```python
from build123d import *

# Parameters (mm, degrees)
IZIM1_R                     = 2
Y_KSEKLIK_EKSTR_ZYON1_DEPTH = 2.5
KES_EKSTR_ZYON1_START       = -2.5
IZIM2_R                     = 2
KES_EKSTR_ZYON1_DEPTH       = 2.5


with BuildPart() as part:
    # Çizim1 → Yükseklik-Ekstrüzyon1 (new, symmetric)
    with BuildSketch(Plane(origin=(0, 0, 0), x_dir=(1, 0, 0), z_dir=(0, 1, 0))):
        with BuildLine():
            Line((-45, 7), (45, 7))
            ThreePointArc((45, 7), (52, 0), (45, -7))
            Line((45, -7), (-45, -7))
            ThreePointArc((-45, -7), (-52, 0), (-45, 7))
        make_face()
        with Locations(Location((-45, 0, 0), (0, 0, 270))):
            Circle(IZIM1_R, mode=Mode.SUBTRACT)
        with Locations(Location((45, 0, 0), (0, 0, 270))):
            Circle(IZIM1_R, mode=Mode.SUBTRACT)
    extrude(amount=Y_KSEKLIK_EKSTR_ZYON1_DEPTH, both=True)

    # Çizim2 → Kes-Ekstrüzyon1 (cut)
    with BuildSketch(Plane.XZ.offset(2.5).offset(KES_EKSTR_ZYON1_START)):
        with Locations(Location((0, 0, 0), (0, 0, 270))):
            Circle(IZIM2_R)
    extrude(amount=KES_EKSTR_ZYON1_DEPTH, mode=Mode.SUBTRACT)


solid = part.part
```
For this review, take the finished solid that the model builds, in its own axes (mm). A direction names the side the tool comes from. Round coordinates to 2 decimals unless told otherwise and drop trailing zeros. Write each loop counter-clockwise with the first axis right and the second up, starting at its lowest first coordinate (ties: lowest second). Pieces come first, ordered by that corner, then holes. Notation, with made-up numbers: (24.5, 86) -> (42.5, 86) arc R26 cw to (42.5, 113) -> close; hole circle Ø4 at (18.25, -7.5). An arc over 180 degrees is marked (long way). Use one line per item in the form item = value.
1) Take a section at D-D, the plane z = -5.5. Write out the cut boundary in (x, y), and give its area (3 significant figures).
Found:
outline = (-49.33, -2.5) -> (49.33, -2.5) -> (49.33, 2.5) -> (-49.33, 2.5) -> close
area = 493 mm2
2) Take a section at B-B, the plane y = -1.55. Write out the cut boundary in (x, z).
Found:
outline = (-45, -7) -> (45, -7) arc R7 ccw to (45, 7) -> (-45, 7) arc R7 ccw to start; hole circle Ø4 at (-45, 0); hole circle Ø4 at (0, 0); hole circle Ø4 at (45, 0)
3) Take a section at A-A, the plane z = 0. Write out the cut boundary in (x, y), and give its area (3 significant figures).
Found:
outline = (-52, -2.5) -> (-47, -2.5) -> (-47, 2.5) -> (-52, 2.5) -> close; (-43, -2.5) -> (-2, -2.5) -> (-2, 0) -> (2, 0) -> (2, -2.5) -> (43, -2.5) -> (43, 2.5) -> (-43, 2.5) -> close; (47, -2.5) -> (52, -2.5) -> (52, 2.5) -> (47, 2.5) -> close
area = 470 mm2
4) To check wall thickness, follow L1, parallel to X at y = 1, z = 0; L2, parallel to X at y = -0.7, z = 0; L3, parallel to Y at x = -1.5, z = 1. State the ranges of each line that lie inside material, in increasing order. Write a range as from..to.
Found:
L1 = -52..-47, -43..43, 47..52
L2 = -52..-47, -43..-2, 2..43, 47..52
L3 = 0..2.5
5) Mouldability with a two-part tool opening along Z and no side actions: class faces 3 (the cylindrical face through (43, 0, 0)), 4 (the flat face through (-1, 0, -7)), 5 (the flat face through (1, 0, 7)) as +Z half, -Z half, draft (parallel to the pull), parting line (faces both ways), or undercut.
Found:
face_3 = undercut
face_4 = -Z half
face_5 = +Z half
6) Take a section at C-C, the plane x = 0. Write out the cut boundary in (y, z), and give its area (3 significant figures).
Found:
outline = (-2.5, -7) -> (2.5, -7) -> (2.5, 7) -> (-2.5, 7) -> (-2.5, 2) -> (0, 2) -> (0, -2) -> (-2.5, -2) -> close
area = 60.0 mm2
7) Tool access review of faces 1 (the cylindrical face through (-2, -1, 0)), 2 (the flat face through (1, 2.5, 0)): name each direction out of +Z, -Z, +X, -X, +Y, -Y from which nothing blocks a thin tool from reaching the whole face with its end or side.
Found:
face_1 = -Y
face_2 = +Z, -Z, +X, -X, +Y
